Verification items for this drawing (mm, ordinates from the low corner). A direction names the side the tool comes from. Give positions to 0.01 mm unless a question says otherwise; leave off trailing zeros. Order: outer loops, then holes, each group sorted by start corner. A loop starts at its lowest first (then second) coordinate and runs counter-clockwise, first axis right, second up.
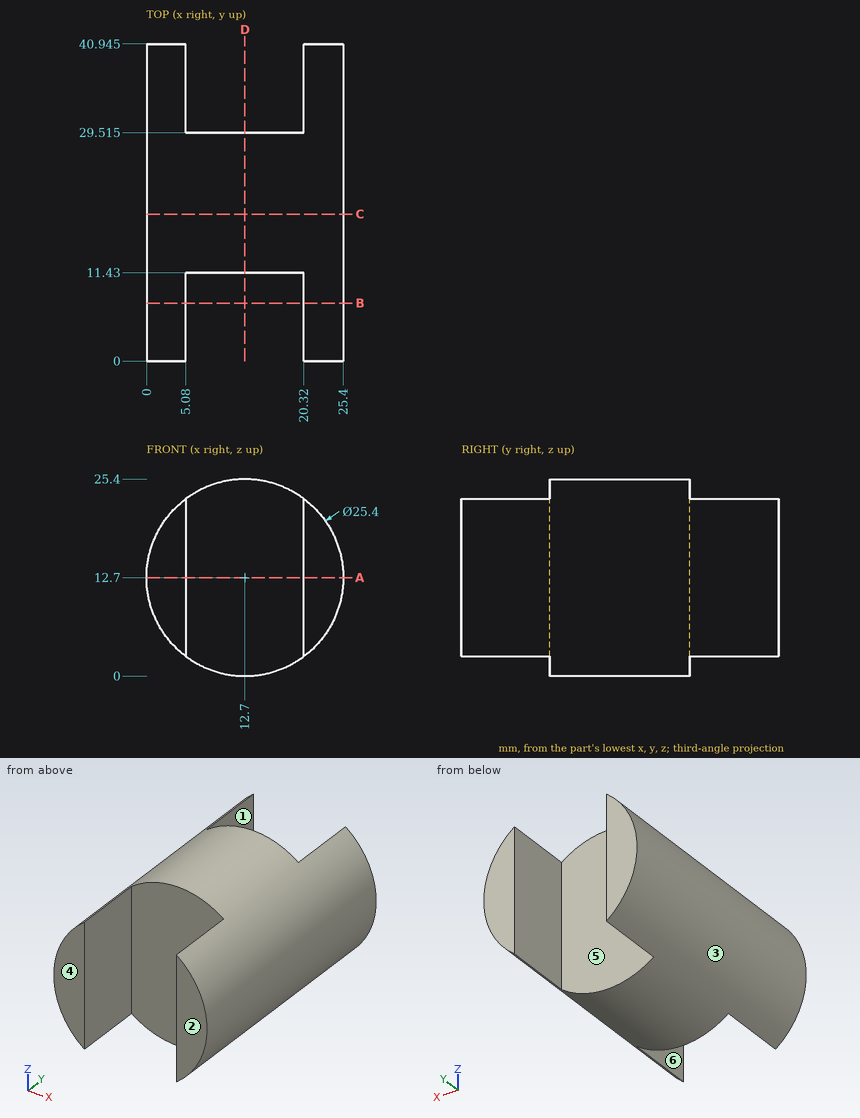
Q1. Cross-section at A-A, the plane z = 12.7. Record the boundary of the cut face in (x, y) (1 decimal).
Q2. Release check for a two-part mould opening along X. For the marked faces 1, 2 and 3 record: pulls with the +X half, pulls with the -X half, needs draft (parallel to the pull), parting line crosses it, or undercut.
Q3. Thickness scan on L1, parallel to X at y = 2, z = 12.5; L2, parallel to X at y = 11, z = 21.75; L3, parallel to Y at x = 8.25, z = 8 (1 decimal). Record the ranges inside material, lowest first.
Q4. Gauge pin test, flat ends, axial feed: P1, Ø1.5, axis at x = 15.5, y = 11.5, coming from the -Z side; P2, Ø5.5, axis at y = 34, z = 17.5, coming from the +X side; P3, Ø2, axis at y = 15.5, z = 22.5, coming from the -X side. Record the tip position at first contact, or that the pin passes through.
Q5. Access from +Z, -Z, +X, -X, +Y, -Y to the whole of each face (thin tool, end or side, straight path). Record for the marked faces 4, 5 and 6.
Q6. Cross-section at D-D, the plane x = 12.7. Record the boundary of the cut face in (y, z) (1 decimal), and give its area (3 significant figures).
Q7. Cross-section at B-B, the plane y = 7.5. Record the boundary of the cut face in (x, z).
Q8. Cross-section at C-C, the plane y = 19. Record the boundary of the cut face in (x, z), and give its area (3 significant figures).
Answers follow:
1. outline: (0, 0) - (5.1, 0) - (5.1, 11.4) - (20.3, 11.4) - (20.3, 0) - (25.4, 0) - (25.4, 40.9) - (20.3, 40.9) - (20.3, 29.5) - (5.1, 29.5) - (5.1, 40.9) - (0, 40.9) - close
2. face 1: undercut
2. face 2: needs draft
2. face 3: parting line crosses it
3. L1: x = 0 to 5.08, 20.32 to 25.4
3. L2: x = 3.79 to 5.08, 20.32 to 21.61
3. L3: y = 11.4 to 29.5
4. P1: stops at z = 0.17
4. P2: stops at x = 25.23
4. P3: stops at x = 3.54
5. face 4: +Z, -Z, +X, -X, -Y
5. face 5: +Z, -Z, +Y
5. face 6: +Z, -Z, -Y
6. outline: (11.4, 0) - (29.5, 0) - (29.5, 25.4) - (11.4, 25.4) - close
6. area: 459 mm2
7. outline: (5.08, 2.54) - (5.08, 22.86) arc R12.7 ccw to start; (20.32, 2.54) arc R12.7 ccw to (20.32, 22.86) - close
8. outline: circle Ø25.4 at (12.7, 12.7)
8. area: 507 mm2
